For this review, take the finished solid that the model builds, in its own axes (mm). A direction names the side the tool comes from. Give positions to 0.01 mm unless a question says otherwise; leave off trailing zeros. Loops run counter-clockwise (first coordinate to the right, second up) from the corner with the lowest first, then second, coordinate; pieces in that order, holes last. Notation, with made-up numbers: (-18.75, 84.5) - (-14.75, 84.5) arc R22 ccw to (-14.75, 116.5) - close; hole circle Ø1 at (25, 37.25). An arc over 180 degrees is marked (long way). Put each result on its own line as item: value.
from build123d import *

# Parameters (mm, degrees)
F0_W     = 596.9
F0_H     = 635
F1_DEPTH = 876.3
F6_W     = 69.85
F6_H     = 101.6
F7_DEPTH = 596.9010001


with BuildPart() as f1:
    # F0 (on Top) → F1 (new body)
    with BuildSketch(Plane.XY):
        Rectangle(F0_W, F0_H)
    extrude(amount=-F1_DEPTH)

    # F5: sweep along a path in F3
    with BuildLine(Plane.XY.offset(-152.4)) as f5_path:
        ThreePointArc((-222.25, -317.5), (23.6275020738, -368.1472825465), (263.7350157491, -294.8719447302))
    # F4 (on face) → F5 (sweep)
    with BuildSketch(Plane.XZ.offset(317.5)):
        with BuildLine():
            add(Edge.make_bspline(
                [(-222.25, -130.175), (-244.2470452561, -130.175), (-233.2485226281, -163.5125), (-222.25, -196.85), (-211.2514773719, -163.5125), (-200.2529547439, -130.175), (-222.25, -130.175)],
                knots=[0, 0, 0, 2.0943951024, 2.0943951024, 4.1887902048, 4.1887902048, 6.2831853072, 6.2831853072, 6.2831853072], degree=2, weights=[1, 0.5, 1, 0.5, 1, 0.5, 1]))
        make_face()
    sweep(path=f5_path.line)

    # F6 (on face) → F7 (cut, through all)
    with BuildSketch(Plane.YZ.offset(298.45)):
        with Locations((-282.575, -825.5)):
            Rectangle(F6_W, F6_H)
    extrude(amount=-F7_DEPTH, mode=Mode.SUBTRACT)


solid = f1.part
1) Take a section at B-B on z = -377.5. State the section outline as (x, y) points, and give its area (3 significant figures).
Geometry check:
outline: (-298.45, -317.5) - (298.45, -317.5) - (298.45, 317.5) - (-298.45, 317.5) - close
area: 379,000 mm²
2) Insertion check: pin 1 Ø8 at (x, z) = (-165.5, -264.5) entering from -Y. The pin has a flat end and moves straight along its axis. Give the tip position at first contact, or say it passes through.
Geometry check:
pin 1: stops at y = -317.5
3) Take a section at C-C on x = -262. State the section outline as (y, z) points, and give its area (3 significant figures).
Geometry check:
outline: (-317.5, -774.7) - (-247.65, -774.7) - (-247.65, -876.3) - (317.5, -876.3) - (317.5, 0) - (-317.5, 0) - close
area: 549,000 mm²
4) For faces 1 (the face through (4, -247.65, -826)), 2 (the face through (-4, 39, -876.3)), list the 3-axis set-ups (+Z, -Z, +X, -X, +Y, -Y) from which the entire face can be reached by the end or side of a thin tool; tool diameter is ignored.
Geometry check:
face 1: -Z, +X, -X, -Y
face 2: -Z, +X, -X, +Y, -Y
5) Take a section at A-A on y = -267. State the section outline as (x, z) points, and give its area (3 significant figures).
Geometry check:
outline: (-298.45, -774.7) - (298.45, -774.7) - (298.45, 0) - (-298.45, 0) - close
area: 462,000 mm²
6) Wall thickness on line 1 (Y direction, x = 30, z = -653.5); line 2 (Y direction, x = 124.5, z = -132); line 3 (Z direction, x = -156, y = -248): over which ranges is each line inside the solid? List them lowest first.
Geometry check:
line 1: y = -317.5 to 317.5
line 2: y = -355.5 to -350.95, -317.5 to 317.5
line 3: z = -774.7 to 0
